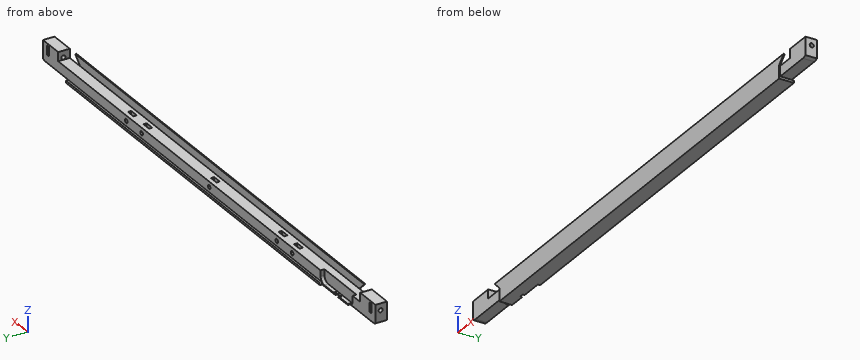
```python
from build123d import *

# Parameters (mm, degrees)
BOSS_EXTRUDE1_DEPTH = 8
SKETCH2_W           = 22.44
SKETCH2_H           = 10.3
CUT_EXTRUDE1_DEPTH  = 0.6
SKETCH3_W           = 24.44
SKETCH3_H           = 10.3
CUT_EXTRUDE2_DEPTH  = 0.6
BOSS_EXTRUDE2_DEPTH = 0.6
SKETCH5_R           = 1.1
CUT_EXTRUDE3_DEPTH  = 296.386661852
CUT_EXTRUDE4_START  = -3.6
CUT_EXTRUDE4_DEPTH  = 1.8
CUT_EXTRUDE5_START  = -3.6
CUT_EXTRUDE5_DEPTH  = 1.8
SKETCH8_W           = 295.2
SKETCH8_H           = 10.4
CUT_EXTRUDE6_DEPTH  = 1.2
CUT_EXTRUDE7_START  = -2.4
CUT_EXTRUDE7_DEPTH  = 1.8
SKETCH10_R          = 1.1
CUT_EXTRUDE8_DEPTH  = 5
SKETCH11_W          = 5
SKETCH11_H          = 2.2
CUT_EXTRUDE9_DEPTH  = 0.2
SKETCH12_W          = 2.2
SKETCH12_H          = 2.2
CUT_EXTRUDE10_DEPTH = 0.2
CUT_EXTRUDE11_DEPTH = 1.2
CUT_EXTRUDE12_DEPTH = 2.1
CUT_EXTRUDE13_START = 1.1
SKETCH15_R          = 5.6
CUT_EXTRUDE13_DEPTH = 1


with BuildPart() as part:
    # Sketch1 → Boss-Extrude1 (new body)
    with BuildSketch(Plane(origin=(0, 0, 0), x_dir=(1, 0, 0), z_dir=(0, 1, 0))):
        with BuildLine():
            Line((-134.1, 0), (134.1, 0))
            Line((134.1, 0), (134.1, -4.8))
            Line((134.1, -4.8), (147.6, -4.8))
            Line((147.6, -4.8), (147.6, 4.898780306))
            ThreePointArc((147.6, 4.898780306), (146.488640518, 5.347211642), (145.3, 5.5))
            Line((145.3, 5.5), (125.16, 5.5))
            Line((125.16, 5.5), (125.16, 6.8))
            Line((125.16, 6.8), (-123.16, 6.8))
            Line((-123.16, 6.8), (-123.16, 5.5))
            Line((-123.16, 5.5), (-145.3, 5.5))
            ThreePointArc((-145.3, 5.5), (-146.488640518, 5.347211642), (-147.6, 4.898780306))
            Line((-147.6, 4.898780306), (-147.6, -4.8))
            Line((-147.6, -4.8), (-134.1, -4.8))
            Line((-134.1, -4.8), (-134.1, 0))
        make_face()
    extrude(amount=BOSS_EXTRUDE1_DEPTH)

    # Sketch2 → Cut-Extrude1 (cut)
    with BuildSketch(Plane.XZ):
        with Locations((136.38, -0.35)):
            Rectangle(SKETCH2_W, SKETCH2_H)
    extrude(amount=-CUT_EXTRUDE1_DEPTH, mode=Mode.SUBTRACT)

    # Sketch3 → Cut-Extrude2 (cut)
    with BuildSketch(Plane.XZ):
        with Locations((-135.38, -0.35)):
            Rectangle(SKETCH3_W, SKETCH3_H)
    extrude(amount=-CUT_EXTRUDE2_DEPTH, mode=Mode.SUBTRACT)

    # Sketch4 → Boss-Extrude2 (add)
    with BuildSketch(Plane.XZ):
        Polygon((129.318578644, 4.3), (125.16, 0.141421356), (125.16, 0), (-123.16, 0), (-123.16, 0.141421356), (-127.318578644, 4.3), align=None)
    extrude(amount=-BOSS_EXTRUDE2_DEPTH)

    # Sketch5 → Cut-Extrude3 (cut, through all)
    with BuildSketch(Plane(origin=(147.6, 0, 0), x_dir=(0, 0, -1), z_dir=(1, 0, 0))):
        with Locations((-1.2, 4)):
            Circle(SKETCH5_R)
    extrude(amount=-CUT_EXTRUDE3_DEPTH, mode=Mode.SUBTRACT)

    # Sketch6 → Cut-Extrude4 (cut)
    with BuildSketch(Plane(origin=(147.6, 0, 0), x_dir=(0, 0, -1), z_dir=(1, 0, 0)).offset(CUT_EXTRUDE4_START)):
        Polygon((-3.7, 5.443375673), (-3.7, 8), (1.3, 8), (1.3, 5.443375673), (1.3, 2.556624327), (-1.2, 1.113248654), (-3.7, 2.556624327), align=None)
    extrude(amount=-CUT_EXTRUDE4_DEPTH, mode=Mode.SUBTRACT)

    # Sketch7 → Cut-Extrude5 (cut)
    with BuildSketch(Plane.ZY.offset(147.6).offset(CUT_EXTRUDE5_START)):
        Polygon((-1.3, 8), (-1.3, 2.556624327), (1.2, 1.113248654), (3.7, 2.556624327), (3.7, 8), align=None)
    extrude(amount=-CUT_EXTRUDE5_DEPTH, mode=Mode.SUBTRACT)

    # Sketch8 → Cut-Extrude6 (cut)
    with BuildSketch(Plane(origin=(0, 8, 0), x_dir=(1, 0, 0), z_dir=(0, 1, 0))):
        with Locations((0, 0.4)):
            Rectangle(SKETCH8_W, SKETCH8_H)
    extrude(amount=-CUT_EXTRUDE6_DEPTH, mode=Mode.SUBTRACT)

    # Sketch9 → Cut-Extrude7 (cut)
    with BuildSketch(Plane(origin=(0, 6.8, 0), x_dir=(1, 0, 0), z_dir=(0, 1, 0)).offset(CUT_EXTRUDE7_START)):
        Polygon((-71.2, 1.456624327), (-71.2, 4.343375673), (-73.7, 5.786751346), (-76.2, 4.343375673), (-76.2, 1.456624327), (-76.2, 0), (-71.2, 0), align=None)
        Polygon((76.2, 1.456624327), (76.2, 4.343375673), (73.7, 5.786751346), (71.2, 4.343375673), (71.2, 1.456624327), (71.2, 0), (76.2, 0), align=None)
        Polygon((-57.5, 1.456624327), (-57.5, 4.343375673), (-60, 5.786751346), (-62.5, 4.343375673), (-62.5, 1.456624327), (-62.5, 0), (-57.5, 0), align=None)
        Polygon((2.5, 1.456624327), (2.5, 4.343375673), (0, 5.786751346), (-2.5, 4.343375673), (-2.5, 1.456624327), (-2.5, 0), (2.5, 0), align=None)
        Polygon((62.5, 1.456624327), (62.5, 4.343375673), (60, 5.786751346), (57.5, 4.343375673), (57.5, 1.456624327), (57.5, 0), (62.5, 0), align=None)
    extrude(amount=-CUT_EXTRUDE7_DEPTH, mode=Mode.SUBTRACT)

    # Sketch10 → Cut-Extrude8 (cut)
    with BuildSketch(Plane(origin=(0, 6.8, 0), x_dir=(1, 0, 0), z_dir=(0, 1, 0))):
        with Locations(Location((-73.7, 2.9, 0), (0, 0, 270))):
            Circle(SKETCH10_R)
        with Locations(Location((73.7, 2.9, 0), (0, 0, 270))):
            Circle(SKETCH10_R)
        with Locations(Location((60, 2.9, 0), (0, 0, 270))):
            Circle(SKETCH10_R)
        with Locations(Location((0, 2.9, 0), (0, 0, 270))):
            Circle(SKETCH10_R)
        with Locations(Location((-60, 2.9, 0), (0, 0, 270))):
            Circle(SKETCH10_R)
    extrude(amount=-CUT_EXTRUDE8_DEPTH, mode=Mode.SUBTRACT)

    # Sketch11 → Cut-Extrude9 (cut)
    with BuildSketch(Plane.XZ.offset(-4.4)):
        with Locations((73.7, -2.9)):
            Rectangle(SKETCH11_W, SKETCH11_H)
        with Locations((60, -2.9)):
            Rectangle(SKETCH11_W, SKETCH11_H)
        with Locations((0, -2.9)):
            Rectangle(SKETCH11_W, SKETCH11_H)
        with Locations((-60, -2.9)):
            Rectangle(SKETCH11_W, SKETCH11_H)
        with Locations((-73.7, -2.9)):
            Rectangle(SKETCH11_W, SKETCH11_H)
    extrude(amount=-CUT_EXTRUDE9_DEPTH, mode=Mode.SUBTRACT)

    # Sketch12 → Cut-Extrude10 (cut)
    with BuildSketch(Plane(origin=(0, 4.6, 0), x_dir=(-1, 0, 0), z_dir=(0, -1, 0))):
        with Locations((73.7, 2.9)):
            Rectangle(SKETCH12_W, SKETCH12_H)
        with Locations((60, 2.9)):
            Rectangle(SKETCH12_W, SKETCH12_H)
        with Locations((0, 2.9)):
            Rectangle(SKETCH12_W, SKETCH12_H)
        with Locations((-60, 2.9)):
            Rectangle(SKETCH12_W, SKETCH12_H)
        with Locations((-73.7, 2.9)):
            Rectangle(SKETCH12_W, SKETCH12_H)
    extrude(amount=-CUT_EXTRUDE10_DEPTH, mode=Mode.SUBTRACT)

    # Sketch13 → Cut-Extrude11 (cut)
    with BuildSketch(Plane(origin=(0, 8, 0), x_dir=(1, 0, 0), z_dir=(0, 1, 0))):
        with BuildLine():
            Line((-100.3, 6.8), (-123.16, 6.8))
            Line((-123.16, 6.8), (-123.16, 5.5))
            Line((-123.16, 5.5), (-99.1, 5.6))
            ThreePointArc((-99.1, 5.6), (-99.948528137, 5.951471863), (-100.3, 6.8))
        make_face()
    extrude(amount=-CUT_EXTRUDE11_DEPTH, mode=Mode.SUBTRACT)

    # Sketch14 → Cut-Extrude12 (cut)
    with BuildSketch(Plane(origin=(0, 6.8, 0), x_dir=(1, 0, 0), z_dir=(0, 1, 0))):
        with BuildLine():
            Line((-98.9, 0), (-127.3, 0))
            Line((-127.3, 0), (-127.3, 2.9))
            add(Edge.make_bspline(
                [(-123.9, 6.2), (-127.3, 6.2), (-127.3, 2.9)],
                knots=[4.71238898, 4.71238898, 4.71238898, 6.283185307, 6.283185307, 6.283185307], degree=2, weights=[1, 0.707106781, 1]))
            Line((-123.9, 6.2), (-102.1, 6.2))
            add(Edge.make_bspline(
                [(-98.9, 3.1), (-98.9, 6.2), (-102.1, 6.2)],
                knots=[3.141592654, 3.141592654, 3.141592654, 4.71238898, 4.71238898, 4.71238898], degree=2, weights=[1, 0.707106781, 1]))
            Line((-98.9, 3.1), (-98.9, 0))
        make_face()
    extrude(amount=-CUT_EXTRUDE12_DEPTH, mode=Mode.SUBTRACT)

    # Sketch15 → Cut-Extrude13 (cut)
    with BuildSketch(Plane(origin=(0, 4.7, 0), x_dir=(1, 0, 0), z_dir=(0, 1, 0)).offset(CUT_EXTRUDE13_START)):
        with Locations((-113.1, 1.3)):
            Circle(SKETCH15_R)
    extrude(amount=CUT_EXTRUDE13_DEPTH, mode=Mode.SUBTRACT)


solid = part.part
```
The listing builds one solid part. Answer for the finished solid, in the listing's coordinates (mm). Coordinates: 2 decimals unless noted, no trailing zeros. Write each loop counter-clockwise with the first axis right and the second up, starting at its lowest first coordinate (ties: lowest second). Pieces come first, ordered by that corner, then holes. Notation, with made-up numbers: (11, 20) - (16, 20) arc R8 cw to (16, 33) - close; hole circle Ø2 at (63, 84). An arc over 180 degrees is marked (long way). Return JSON: item names as keys, results as strings. Group by question number.
1. Given pin 1 (3 mm diameter, centred on x = 73.7, z = -2.9, fed in from +Y); pin 2 (1.9 mm diameter, centred on x = -112.5, z = -2.5, fed in from +Y), each flat-ended and moving along its own axis, determine where each tip first touches the part or whether it passes through.
2. A cutting plane is placed at A-A, the plane x = 25. Determine the outline of the cut face in (y, z), plus the area to 3 significant figures.
3. Straight lines are drawn through the part: L1, parallel to X at y = 1.75, z = 1.75; L2, parallel to X at y = 2.1, z = -2.9; L3, parallel to Y at x = -146.3, z = 1.2. For each, find the intervals that lie inside material, in ascending order.
Ans:
{
 "1": {"pin 1": "y = 6.8", "pin 2": "y = 4.7"},
 "2": {"outline": "(0, -6.8) - (8, -6.8) - (8, -5.6) - (6.8, -5.6) - (6.8, 0) - (0.6, 0) - (0.6, 4.3) - (0, 4.3) - close", "area": "50.3 mm²"},
 "3": {"L1": "-147.6 to -144, -142.2 to -134.1, 134.1 to 142.2, 144 to 147.6", "L2": "-147.6 to -74.8, -72.6 to -61.1, -58.9 to -1.1, 1.1 to 58.9, 61.1 to 72.6, 74.8 to 147.6", "L3": "0.6 to 2.9, 5.1 to 6.8"}
}
